Geometry: see drawing. Coordinates: mm, zero at the bounding-box minimum. A direction names the side the tool comes from. Coordinates: 2 decimals unless noted, no trailing zeros. Write each loop counter-clockwise with the first axis right and the second up, starting at its lowest first coordinate (ties: lowest second). Pieces come first, ordered by that corner, then holes.
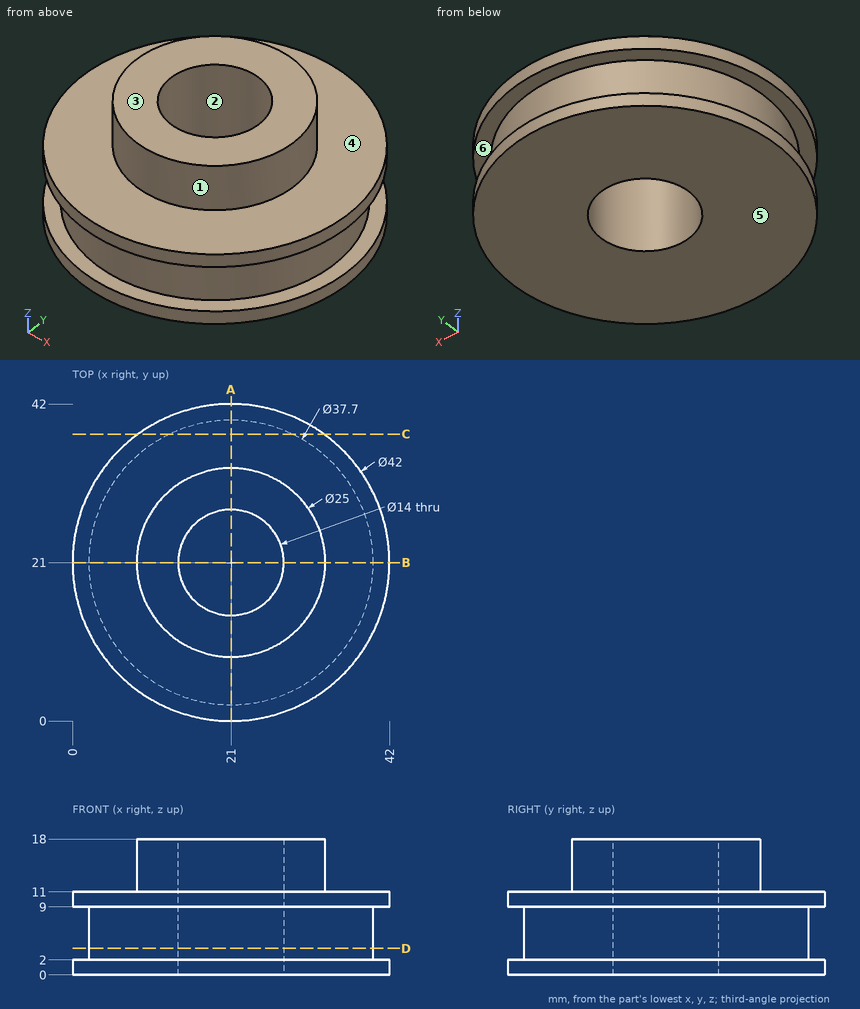
Item 1: Pin query (flat end, axial travel): pin 1 (1 mm diameter, centred on x = 6, z = 12, fed in from +Y); pin 2 (8 mm diameter, centred on x = 19, z = 2, fed in from +Y); pin 3 (2 mm diameter, centred on x = 28, z = 8.5, fed in from +Y); pin 4 (2 mm diameter, centred on y = 14.5, z = 5.5, fed in from +X). Return the tip coordinate at first contact, or that it passes through.
Derived:
pin 1: passes through
pin 2: stops at y = 42
pin 3: stops at y = 41.08
pin 4: stops at x = 39.03
Item 2: Section A-A, the plane x = 21. Output: boundary loops of the cut face in (y, z).
Derived:
outline: (0, 0) - (14, 0) - (14, 18) - (8.5, 18) - (8.5, 11) - (0, 11) - (0, 9) - (2.15, 9) - (2.15, 2) - (0, 2) - close; (28, 0) - (42, 0) - (42, 2) - (39.85, 2) - (39.85, 9) - (42, 9) - (42, 11) - (33.5, 11) - (33.5, 18) - (28, 18) - close
Item 3: Section C-C, the plane y = 38. Output: boundary loops of the cut face in (x, z), plus the area to 3 significant figures.
Derived:
outline: (8.67, 0) - (33.33, 0) - (33.33, 2) - (29.14, 2) - (29.14, 9) - (33.33, 9) - (33.33, 11) - (8.67, 11) - (8.67, 9) - (12.86, 9) - (12.86, 2) - (8.67, 2) - close
area: 213 mm2
Item 4: Pull-direction query (X, two-part tool) for the marked faces 1, 2 and 3; classes: released by +X, released by -X, zero draft, split by the parting line, or undercut.
Derived:
face 1: split by the parting line
face 2: undercut
face 3: zero draft
Item 5: Set-up query: the marked faces 4, 5 and 6. Return all of +Z, -Z, +X, -X, +Y, -Y with unobstructed straight access to the full face (end or side cutting, diameter ignored); none if empty.
Derived:
face 4: +Z
face 5: -Z, +X, -X, +Y, -Y
face 6: none
Item 6: Section D-D, the plane z = 3.5. Output: boundary loops of the cut face in (x, y), plus the area to 3 significant figures.
Derived:
outline: circle Ø37.7 at (21, 21); hole circle Ø14 at (21, 21)
area: 962 mm2
Item 7: Material intervals for probe 1 along Z at (x, y) = (30, 4); probe 2 along Y at (x, z) = (21, 13.25); probe 3 along Y at (x, z) = (21, 7.5), sorted ascending.
Derived:
probe 1: z = 0 to 2, 9 to 11
probe 2: y = 8.5 to 14, 28 to 33.5
probe 3: y = 2.15 to 14, 28 to 39.85
